Input: part model. Units: mm. Frame: model coordinates. Coordinates: 2 decimals unless noted, no trailing zeros. Write each loop counter-clockwise with the first axis right and the second up, starting at its lowest first coordinate (ties: lowest second). Pieces come first, ordered by that corner, then holes. Notation, with made-up numbers: M -34.5,18 L -22.5,18 A23 ccw -22.5,29 Z; hole C -4,19 d11. An arc over 180 degrees is marked long. Write each question's results on one line, items separated by ' | '. Start each with the question number.
1. Section query C-C, the plane x = 61. Output: boundary loops of the cut face in (y, z), and give its area (3 significant figures).
2. First-contact query: pin 1 (0.9 mm diameter, centred on x = 6.35, y = 19.05, fed in from -Z). Flat tip, straight axial feed; report the tip coordinate or a pass-through.
3. Section query A-A, the plane z = 0.75. Output: boundary loops of the cut face in (x, y), and give its area (3 significant figures).
4. Ray query, probe 1 along Y at (x, z) = (6.35, 1.5); probe 2 along X at (y, z) = (18.75, 1.1); probe 3 along Y at (x, z) = (101, 2). Return the intervals inside material, ascending.
5. Section query B-B, the plane x = 73. Output: boundary loops of the cut face in (y, z), and give its area (3 significant figures).
```python
from build123d import *

# Parameters (mm, degrees)
F1_DEPTH = 2.54
F2_R     = 0.73531
F3_DEPTH = 25.4


with BuildPart() as f1:
    # F0 (on Top) → F1 (new body)
    with BuildSketch(Plane.XY):
        with BuildLine():
            Line((0, 25.4), (0, 0))
            Line((0, 0), (43.18, 0))
            Line((43.18, 0), (111.666013, 3.5892))
            ThreePointArc((111.666013, 3.5892), (119.286013, 12.7), (111.666013, 21.8108))
            Line((111.666013, 21.8108), (43.18, 25.4))
            Line((43.18, 25.4), (0, 25.4))
        make_face()
    extrude(amount=F1_DEPTH)

    # F2 (on face) → F3 (cut)
    with BuildSketch(Plane.XY.offset(2.54)):
        with Locations((6.35, 19.05)):
            Circle(F2_R)
        with Locations((6.35, 6.35)):
            Circle(F2_R)
        with Locations((38.1, 6.35)):
            Circle(F2_R)
        with Locations((38.1, 19.05)):
            Circle(F2_R)
    extrude(amount=-F3_DEPTH, mode=Mode.SUBTRACT)


solid = f1.part
```
Answer:
1) outline: M 0.93,0 L 24.47,0 L 24.47,2.54 L 0.93,2.54 Z | area: 59.8 mm^2
2) pin 1: through
3) outline: M 0,0 L 43.18,0 L 111.67,3.59 A9.26 ccw 111.67,21.81 L 43.18,25.4 L 0,25.4 Z; hole C 6.35,6.35 d1.47; hole C 6.35,19.05 d1.47; hole C 38.1,6.35 d1.47; hole C 38.1,19.05 d1.47 | area: 2,690 mm^2
4) probe 1: 0 to 5.61, 7.09 to 18.31, 19.79 to 25.4 | probe 2: 0 to 5.68, 7.02 to 37.43, 38.77 to 117.04 | probe 3: 3.03 to 22.37
5) outline: M 1.56,0 L 23.84,0 L 23.84,2.54 L 1.56,2.54 Z | area: 56.6 mm^2
